Read the model definition and answer for the solid it produces. Units are mm, in the model's axes. A direction names the side the tool comes from. Coordinates: 2 decimals unless noted, no trailing zeros. Write each loop counter-clockwise with the first axis right and the second up, starting at its lowest first coordinate (ties: lowest second). Pieces come first, ordered by that corner, then holes. Notation, with made-up numbers: (56, 3.5) -> (76, 3.5) arc R22 ccw to (76, 11.5) -> close; hole circle Ø9 at (87.25, 57.25). An arc over 180 degrees is marked (long way). Answer as a JSON object with one key per item and string values. Group by question number.
(1) Find section C-C (x = -13). Give the vertices of the cut face in (y, z).
(2) Find section B-B (y = -12.5). Give the vertices of the cut face in (x, z), then the cut area to 3 significant figures.
(3) Straight lines are drawn through the part: L1, parallel to Z at x = -3.5, y = -7.75; L2, parallel to Y at x = -2, z = 78; L3, parallel to Y at x = -12, z = 182.5. For each, find the intervals that lie inside material, in ascending order.
(4) Flat-ended cylindrical pins translate along their axes: P1, Ø5, axis at y = -3, z = 120.5, coming from the -X side; P2, Ø4, axis at y = -10.5, z = 114, coming from the -X side. Find the tip coordinate at first contact, or state that the pin passes through.
(5) Find section A-A (z = 117.5). Give the vertices of the cut face in (x, y), then the cut area to 3 significant figures.
(6) Which of the six approach directions +Z, -Z, +X, -X, +Y, -Y give full straight-line access (tool end or side, diameter ignored) to faces 4 (the face through (0, -10, 106)), 5 (the face through (-6.993, -6.645, 106.453))?
(7) For a pull along Z with two mould halves and no side action, classify faces 1 (the face through (-3.5, -3.07, 106.32)), 2 (the face through (-8, -7, -8.3)), 3 (the face through (-5.72, -5.09, 106.45)) as +Z half, -Z half, draft (parallel to the pull), parting line (faces both ways), or undercut.
from build123d import *

# Parameters (mm, degrees)
BOSS_EXTRUDE1_DEPTH   = 215.9
BOSS_EXTRUDE1_2_DEPTH = 215.9
BOSS_EXTRUDE2_DEPTH   = 8.3
BOSS_EXTRUDE3_START   = 8.3
BOSS_EXTRUDE3_DEPTH   = 8.3
FILLET1_R             = 1


with BuildPart() as part:
    # Sketch1 → Boss-Extrude1 (new body)
    with BuildSketch(Plane.XY):
        with BuildLine():
            Line((-5, 0.503476918), (-8, 0.503476918))
            ThreePointArc((-8, 0.503476918), (-5.656854249, -5.153377331), (0, -7.496523082))
            Line((0, -7.496523082), (0, -4.496523082))
            ThreePointArc((0, -4.496523082), (-3.535533906, -3.032056988), (-5, 0.503476918))
        make_face()
    extrude(amount=BOSS_EXTRUDE1_DEPTH)



with BuildPart() as body_2:
    # Sketch1 → Boss-Extrude1 2 (new body)
    with BuildSketch(Plane.XY):
        with BuildLine():
            Line((-10, 0.503476918), (-15, 0.503476918))
            ThreePointArc((-15, 0.503476918), (-10.606601718, -10.1031248), (0, -14.496523082))
            Line((0, -14.496523082), (0, -9.496523082))
            ThreePointArc((0, -9.496523082), (-7.071067812, -6.567590894), (-10, 0.503476918))
        make_face()
    extrude(amount=BOSS_EXTRUDE1_2_DEPTH)


with BuildPart() as part_1:
    add(part.part)

    add(body_2.part)  # Boss-Extrude2 merges body 2
    # Sketch2 → Boss-Extrude2 (add)
    with BuildSketch(Plane.XY.offset(215.9)):
        with BuildLine():
            Line((-5, 0.503476918), (-15, 0.503476918))
            ThreePointArc((-15, 0.503476918), (-10.606601718, -10.1031248), (0, -14.496523082))
            Line((0, -14.496523082), (0, -4.496523082))
            ThreePointArc((0, -4.496523082), (-3.535533906, -3.032056988), (-5, 0.503476918))
        make_face()
    extrude(amount=BOSS_EXTRUDE2_DEPTH)

    # Sketch3 → Boss-Extrude3 (add)
    with BuildSketch(Plane(origin=(0, 0, 0), x_dir=(-1, 0, 0), z_dir=(0, 0, -1)).offset(BOSS_EXTRUDE3_START)):
        with BuildLine():
            Line((5, 0.503476918), (15, 0.503476918))
            ThreePointArc((15, 0.503476918), (10.606601718, -10.1031248), (0, -14.496523082))
            Line((0, -14.496523082), (0, -4.496523082))
            ThreePointArc((0, -4.496523082), (3.535533906, -3.032056988), (5, 0.503476918))
        make_face()
    extrude(amount=-BOSS_EXTRUDE3_DEPTH)

    # Fillet1
    fillet1_edges = [part_1.edges().sort_by_distance(p)[0] for p in [
        (-5.656854249, -5.153377331, 0),
        (-7.071067812, -6.567590894, 0),
        (-5.656854249, -5.153377331, 215.9),
        (-7.071067812, -6.567590894, 215.9),
    ]]
    fillet(fillet1_edges, radius=FILLET1_R - 0.0001)  # a hair under: the kernel refuses the full size


solid = part_1.part
Results below:
{
 "1": {"outline": "(-6.98, -8.3) -> (0.5, -8.3) -> (0.5, 224.2) -> (-6.98, 224.2) -> close"},
 "2": {"outline": "(-7.48, -8.3) -> (0, -8.3) -> (0, 224.2) -> (-7.48, 224.2) -> close", "area": "1,740 mm2"},
 "3": {"L1": "z = -8.3 to 0, 215.9 to 224.2", "L2": "y = -14.36 to -9.29, -7.24 to -4.08", "L3": "y = -8.5 to 0.5"},
 "4": {"P1": "stops at x = -14.97", "P2": "stops at x = -12"},
 "5": {"outline": "(-15, 0.5) arc R15 ccw to (0, -14.5) -> (0, -9.5) arc R10 cw to (-10, 0.5) -> close; (-8, 0.5) arc R8 ccw to (0, -7.5) -> (0, -4.5) arc R5 cw to (-5, 0.5) -> close", "area": "129 mm2"},
 "6": {"face 4": "+Z, -Z, +X, +Y, -Y", "face 5": "none"},
 "7": {"face 1": "draft", "face 2": "-Z half", "face 3": "undercut"}
}
